from build123d import *

# Parameters (mm, degrees)
F0_R     = 10.65
F0_R_2   = 8.1
F1_DEPTH = 25
F0_R_3   = 6.5
F2_DEPTH = 2.5
F3_DEPTH = 25
F4_SIZE  = 1


with BuildPart() as f1:
    # F0 (on Top) → F1 (new body, symmetric)
    with BuildSketch(Plane.XY):
        Circle(F0_R)
        Circle(F0_R_2, mode=Mode.SUBTRACT)
    extrude(amount=F1_DEPTH, both=True)

    # F0 (on Top) → F2 (join, symmetric)
    with BuildSketch(Plane.XY):
        Circle(F0_R_2)
        Circle(F0_R_3, mode=Mode.SUBTRACT)
    extrude(amount=F2_DEPTH, both=True)

    # F0 (on Top) → F3 (join, symmetric)
    with BuildSketch(Plane.XY):
        Circle(F0_R_3)
    extrude(amount=F3_DEPTH, both=True)

    # F4
    f4_edges = [f1.edges().sort_by_distance(p)[0] for p in [
        (-8.1, 0, -25),
        (-6.5, 0, -25),
        (-8.1, 0, 25),
        (-6.5, 0, 25),
    ]]
    chamfer(f4_edges, length=F4_SIZE)


solid = f1.part
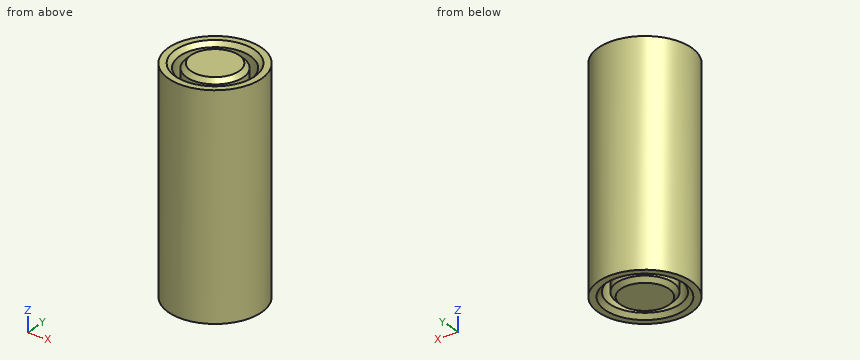
Read the model definition and answer for the solid it produces. Units are mm, in the model's axes. Round coordinates to 2 decimals unless told otherwise and drop trailing zeros. Write each loop counter-clockwise with the first axis right and the second up, starting at its lowest first coordinate (ties: lowest second). Pieces come first, ordered by that corner, then holes.
1. Straight lines are drawn through the part: L1, parallel to Y at x = 0, z = 8; L2, parallel to Y at x = -6, z = 15; L3, parallel to Z at x = 7.5, y = -2.25. For each, find the intervals that lie inside material, in ascending order.
2. The part is cut by section A-A, the plane z = 3.5. Determine the outline of the cut face in (x, y).
3. Given pin 1 Ø10 at (x, z) = (-7.5, -9) entering from -Y; pin 2 Ø6 at (y, z) = (5, -2.5) entering from -X; pin 3 Ø2 at (x, z) = (2.5, 7) entering from +Y; pin 4 Ø8 at (x, y) = (-8, 4) entering from +Z, each flat-ended and moving along its own axis, determine where each tip first touches the part or whether it passes through.
4. The part is cut by section B-B, the plane x = 0. Determine the outline of the cut face in (y, z).
Values:
1. L1: y = -10.65 to -8.1, -6.5 to 6.5, 8.1 to 10.65
1. L2: y = -8.8 to -5.44, -2.5 to 2.5, 5.44 to 8.8
1. L3: z = -2.5 to 2.5
2. outline: circle Ø21.3 at (0, 0); circle Ø13 at (0, 0); hole circle Ø16.2 at (0, 0)
3. pin 1: stops at y = -10.35
3. pin 2: stops at x = -10.46
3. pin 3: stops at y = 10.54
3. pin 4: stops at z = 25
4. outline: (-10.65, -25) - (-9.1, -25) - (-8.1, -24) - (-8.1, -2.5) - (-6.5, -2.5) - (-6.5, -24) - (-5.5, -25) - (5.5, -25) - (6.5, -24) - (6.5, -2.5) - (8.1, -2.5) - (8.1, -24) - (9.1, -25) - (10.65, -25) - (10.65, 25) - (9.1, 25) - (8.1, 24) - (8.1, 2.5) - (6.5, 2.5) - (6.5, 24) - (5.5, 25) - (-5.5, 25) - (-6.5, 24) - (-6.5, 2.5) - (-8.1, 2.5) - (-8.1, 24) - (-9.1, 25) - (-10.65, 25) - close
